Solid Edge part; units mm, degrees
sketch "Sketch1" plane through (0, 0, 0) normal (0, 0, 1) x (1, 0, 0)
  line L0 (-53, -35.5) -> (53, -35.5)
  line L1 (53, -35.5) -> (53, 35.5)
  line L2 (53, 35.5) -> (-53, 35.5)
  line L3 (-53, 35.5) -> (-53, -35.5)
extrude "Protrusion1" add sketch "Sketch1" along normal blind 3
sketch "Sketch2" plane through (0, 0, 3) normal (0, 0, 1) x (0, -1, 0)
  line L0 (-32.4, -49.9) -> (-32.4, 49.9)
  line L1 (-32.4, 49.9) -> (32.4, 49.9)
  line L2 (32.4, 49.9) -> (32.4, -49.9)
  line L3 (32.4, -49.9) -> (-32.4, -49.9)
  line L4 (-29.3, -46.8) -> (-29.3, 46.8)
  line L5 (-29.3, 46.8) -> (29.3, 46.8)
  line L6 (29.3, 46.8) -> (29.3, -46.8)
  line L7 (29.3, -46.8) -> (-29.3, -46.8)
extrude "ExtrudedProtrusion_2" add sketch "Sketch2" along normal blind 5
fillet "Round_1" radius 2 4 edges at (53, -35.5, 1.5) (53, 35.5, 1.5) (-53, 35.5, 1.5) (-53, -35.5, 1.5)
fillet "Round_2" radius 2 8 edges at (49.9, -32.4, 5.5) (49.9, 32.4, 5.5) (-49.9, 32.4, 5.5) (-49.9, -32.4, 5.5) (-46.8, -29.3, 5.5) (46.8, -29.3, 5.5) (46.8, 29.3, 5.5) (-46.8, 29.3, 5.5)
sketch "Sketch3" plane through (0, -32.4, 5.5) normal (0, -1, 0) x (-1, 0, 0)
  line L0 (34.9, 0.75) -> (30.9, 0.75)
  line L1 (30.9, 0.75) -> (30.9, -1.25)
  line L2 (30.9, -1.25) -> (34.9, -1.25)
  line L3 (34.9, -1.25) -> (34.9, 0.75)
  line L4 (-33.1, 0.7516) -> (-29.1, 0.7516)
  line L5 (-29.1, 0.7516) -> (-29.1, -1.2484)
  line L6 (-29.1, -1.2484) -> (-33.1, -1.2484)
  line L7 (-33.1, -1.2484) -> (-33.1, 0.7516)
  dimension "D1" = 30.9
  dimension "D2" = 30.9
extrude "ExtrudedCutout_1" cut sketch "Sketch3" against normal blind 125.4753
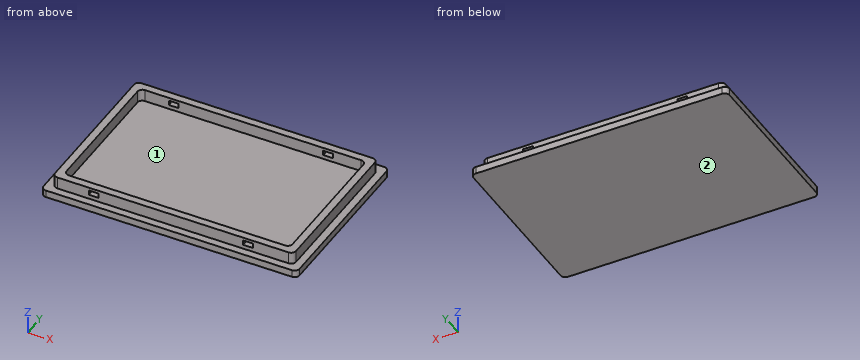
Model file for the job. Use its own axes, mm. Face numbers are marked on the shaded views. Give positions to 0.01 mm unless a question says otherwise; leave off trailing zeros. Loops run counter-clockwise (first coordinate to the right, second up) from the corner with the lowest first, then second, coordinate; pieces in that order, holes last. Notation, with made-up numbers: (65, 13.5) -> (99, 13.5) arc R17 cw to (99, 37.5) -> close; hole circle Ø9 at (3.25, 12). An arc over 180 degrees is marked (long way). Use a Markdown table: item, result. Add a question column.
(1) Mould opens along Y. For the marked faces 1 and 2 say: +Y half, -Y half, draft (parallel to the pull), parting line (faces both ways), or undercut.
(2) Slice it at B-B on y = -8.5. List the corners of the cut face in (x, z), and give its area (3 significant figures).
(3) Wall check: line 1 along Y through (x, z) = (33.5, 6.75); line 2 along X through (y, z) = (-6.5, 3.75); line 3 along Z through (x, y) = (-3.5, 7). Give the ranges that are in metal, low to high.
(4) Slice it at A-A on x = 32. List the corners of the cut face in (y, z), and give its area (3 significant figures).
(5) Drop flat-ended pins along their axis: pin 1 Ø2 at (x, z) = (21.5, 7) entering from +Y; pin 2 Ø2 at (y, z) = (-31, 6) entering from -X; pin 3 Ø0.6 at (y, z) = (30, 6) entering from +X. Give the stop position or say it passes through.
(6) Slice it at C-C on x = -39. List the corners of the cut face in (y, z), and give its area (3 significant figures).
Filled sheet:
| question | item | result |
|---|---|---|
| 1 | face 1 | undercut |
| 1 | face 2 | draft |
| 2 | outline | (-53, 0) -> (53, 0) -> (53, 3) -> (49.9, 3) -> (49.9, 8) -> (46.8, 8) -> (46.8, 3) -> (-46.8, 3) -> (-46.8, 8) -> (-49.9, 8) -> (-49.9, 3) -> (-53, 3) -> close |
| 2 | area | 349 mm2 |
| 3 | line 1 | -32.4 to -29.3, 29.3 to 32.4 |
| 3 | line 2 | -49.9 to -46.8, 46.8 to 49.9 |
| 3 | line 3 | 0 to 3 |
| 4 | outline | (-35.5, 0) -> (35.5, 0) -> (35.5, 3) -> (32.4, 3) -> (32.4, 4.75) -> (29.3, 4.75) -> (29.3, 3) -> (-29.3, 3) -> (-29.3, 4.75) -> (-32.4, 4.75) -> (-32.4, 3) -> (-35.5, 3) -> close; (-32.4, 6.75) -> (-29.3, 6.75) -> (-29.3, 8) -> (-32.4, 8) -> close; (29.3, 6.75) -> (32.4, 6.75) -> (32.4, 8) -> (29.3, 8) -> close |
| 4 | area | 232 mm2 |
| 5 | pin 1 | y = 32.4 |
| 5 | pin 2 | x = -49.9 |
| 5 | pin 3 | x = 49.9 |
| 6 | outline | (-35.5, 0) -> (35.5, 0) -> (35.5, 3) -> (32.4, 3) -> (32.4, 8) -> (29.3, 8) -> (29.3, 3) -> (-29.3, 3) -> (-29.3, 8) -> (-32.4, 8) -> (-32.4, 3) -> (-35.5, 3) -> close |
| 6 | area | 244 mm2 |
